from build123d import *

# Parameters (mm, degrees)
CUT_EXTRUDE_1_DEPTH      = 23.516660498
CUT_EXTRUDE_1_DEPTH_BACK = 23.516660498
SKETCH_2_OUTSIDE_W       = 37.006
SKETCH_2_OUTSIDE_H       = 37.006
SKETCH_2_OUTSIDE_W_2     = 26
SKETCH_2_OUTSIDE_H_2     = 17
CUT_EXTRUDE_2_DEPTH      = 26.039968051
CUT_EXTRUDE_2_DEPTH_BACK = 26.039968051
SKETCH_3_R               = 6
CUT_EXTRUDE_3_DEPTH      = 21.254629101
CUT_EXTRUDE_3_DEPTH_BACK = 21.254629101
SKETCH_4_R               = 2


with BuildPart() as part:
    # 草图1 → 旋转1 (revolve)
    with BuildSketch(Plane(origin=(0, 0, 0), x_dir=(0, 0, -1), z_dir=(1, 0, 0))):
        with BuildLine():
            Line((0, 13), (0, -13))
            ThreePointArc((0, -13), (13, 0), (0, 13))
        make_face()
    revolve(axis=Axis((0, -13, 0), (0, -1, 0)))

    # 草图2 outside → 切除-拉伸1 (cut, two sides: drawn at the far end of the back side and taken through both)
    with BuildSketch(Plane(origin=(0, 0, 0), x_dir=(0, 0, -1), z_dir=(1, 0, 0)).offset(-CUT_EXTRUDE_1_DEPTH_BACK)):
        Rectangle(SKETCH_2_OUTSIDE_W, SKETCH_2_OUTSIDE_H)
        Rectangle(SKETCH_2_OUTSIDE_W_2, SKETCH_2_OUTSIDE_H_2, mode=Mode.SUBTRACT)
    extrude(amount=CUT_EXTRUDE_1_DEPTH + CUT_EXTRUDE_1_DEPTH_BACK, mode=Mode.SUBTRACT)

    # 草图3 → 切除-拉伸2 (cut, two sides: drawn at the far end of the back side and taken through both)
    with BuildSketch(Plane(origin=(0, 8.5, 0), x_dir=(1, 0, 0), z_dir=(0, 1, 0)).offset(-CUT_EXTRUDE_2_DEPTH_BACK)):
        with Locations(Location((0, 0, 0), (0, 0, 270))):
            Circle(SKETCH_3_R)
    extrude(amount=CUT_EXTRUDE_2_DEPTH + CUT_EXTRUDE_2_DEPTH_BACK, mode=Mode.SUBTRACT)

    # 草图4 → 切除-拉伸3 (cut, two sides: drawn at the far end of the back side and taken through both)
    with BuildSketch(Plane(origin=(0, 0, 0), x_dir=(0, 0, -1), z_dir=(1, 0, 0)).offset(-CUT_EXTRUDE_3_DEPTH_BACK)):
        Circle(SKETCH_4_R)
    extrude(amount=CUT_EXTRUDE_3_DEPTH + CUT_EXTRUDE_3_DEPTH_BACK, mode=Mode.SUBTRACT)

    # 草图5 → 旋转2 (revolve)
    with BuildSketch(Plane(origin=(0, 0, 0), x_dir=(0, 0, -1), z_dir=(1, 0, 0))):
        with BuildLine():
            Line((9.925994235, 8.394917417), (98.921294458, 43.451098455))
            ThreePointArc((98.921294458, 43.451098455), (104.361835013, 43.320509784), (108.06465139, 39.332316482))
            Line((108.06465139, 39.332316482), (11.462947931, 4.172171844))
            Line((11.462947931, 4.172171844), (9.925994235, 8.394917417))
        make_face()
    revolve(axis=Axis((0, 4.172171844, -11.462947931), (0, -0.34202014332566955, 0.9396926207859082)))


solid = part.part
Read the model definition and answer for the solid it produces. Units are mm, in the model's axes. Coordinates: 2 decimals unless noted, no trailing zeros. Loops run counter-clockwise (first coordinate to the right, second up) from the corner with the lowest first, then second, coordinate; pieces in that order, holes last.
Q1. The part is cut by section A-A on z = 0. Write down the section's boundary in (x, y), and give its area (3 significant figures).
Q2. Consider probe 1 along Y at (x, z) = (-8.5, 0); probe 2 along Z at (x, y) = (8.75, 0); probe 3 along Z at (x, y) = (10.25, 0). Determine where each line is inside the solid, lowest interval first.
Q3. The part is cut by section C-C on y = -4. Write down the section's boundary in (x, z).
Q4. Each of these flat-tipped pins is pushed along its axis until it touches: pin 1 Ø3 at (x, y) = (9, -1) entering from -Z; pin 2 Ø5 at (x, z) = (-3.5, -65) entering from +Y; pin 3 Ø2.5 at (y, z) = (0, 0) entering from -X; pin 4 Ø12 at (x, z) = (5.5, -8.5) entering from -Y. Where does it stop, or does it pass through?
Q5. The mould has two halves that part along Y. Classify faces 1 (the face through (9, -2, 0)), 2 (the face through (4, -8.5, 5)), 3 (the face through (-9, -2, 0)), 4 (the face through (4, 8.5, 5)): +Y half, -Y half, draft (parallel to the pull), parting line (faces both ways), or undercut.
Q6. The part is cut by section B-B on x = 0. Write down the section's boundary in (y, z).
Results below:
1. outline: (-12.85, -2) arc R13 ccw to (-9.84, -8.5) - (-6, -8.5) - (-6, -2) - close; (-12.85, 2) - (-6, 2) - (-6, 8.5) - (-9.84, 8.5) arc R13 ccw to start; (6, -8.5) - (9.84, -8.5) arc R13 ccw to (12.85, -2) - (6, -2) - close; (6, 2) - (12.85, 2) arc R13 ccw to (9.84, 8.5) - (6, 8.5) - close
1. area: 149 mm2
2. probe 1: y = -8.5 to -2, 2 to 8.5
2. probe 2: z = -9.61 to -2, 2 to 9.61
2. probe 3: z = -8 to -2, 2 to 8
3. outline: circle Ø24.74 at (0, 0); hole circle Ø12 at (0, 0)
4. pin 1: stops at z = -10.58
4. pin 2: stops at y = 30.52
4. pin 3: passes through
4. pin 4: stops at y = -8.5
5. face 1: undercut
5. face 2: -Y half
5. face 3: undercut
5. face 4: +Y half
6. outline: (-8.5, -9.84) arc R13 ccw to (-0.05, -13) - (30.3, -103.71) arc R7 ccw (long way) to (43.45, -98.92) - (8.39, -9.93) arc R13 ccw to (8.5, -9.84) - (8.5, -6) - (-8.5, -6) - close; (-8.5, 6) - (8.5, 6) - (8.5, 9.84) arc R13 ccw to (-8.5, 9.84) - close
